Build history of the part. All positions in model axes, mm. Give positions to 0.01 mm unless a question says otherwise; leave off trailing zeros. Order: outer loops, then holes, each group sorted by start corner. A loop starts at its lowest first (then second) coordinate and runs counter-clockwise, first axis right, second up. Notation, with made-up numbers: M 25.25,-36.5 L 31.25,-36.5 A23 cw 31.25,-4.5 Z; hole C -2,-27 d6. An arc over 180 degrees is marked long. One line per item, written item: value.
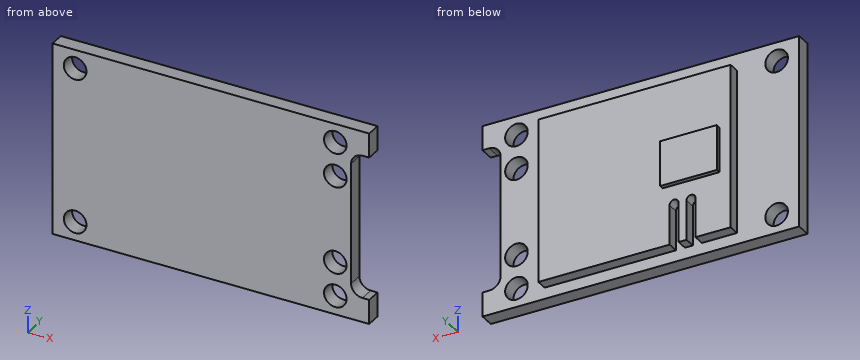
from build123d import *

# Parameters (mm, degrees)
EXTRUDE_1_DEPTH     = 1.3
SKETCH_2_R          = 1
CUT_EXTRUDE_1_DEPTH = 17.429850882
EXTRUDE_2_DEPTH     = 1
SKETCH_4_W          = 5
SKETCH_4_H          = 4
EXTRUDE_3_DEPTH     = 0.4


with BuildPart() as part:
    # Эскиз1 → Бобышка-Вытянуть1 (new body)
    with BuildSketch(Plane(origin=(0, 0, 0), x_dir=(1, 0, 0), z_dir=(0, 1, 0))):
        with BuildLine():
            Line((12.4, 5.35), (12.4, -5.35))
            ThreePointArc((12.4, -5.35), (12.692893219, -6.057106781), (13.4, -6.35))
            Line((13.4, -6.35), (14, -6.35))
            Line((14, -6.35), (14, -8.5))
            Line((14, -8.5), (-14, -8.5))
            Line((-14, -8.5), (-14, 8.5))
            Line((-14, 8.5), (14, 8.5))
            Line((14, 8.5), (14, 6.35))
            Line((14, 6.35), (13.4, 6.35))
            ThreePointArc((13.4, 6.35), (12.692893219, 6.057106781), (12.4, 5.35))
        make_face()
    extrude(amount=EXTRUDE_1_DEPTH)

    # Эскиз2 → Вырез-Вытянуть1 (cut, through all)
    with BuildSketch(Plane(origin=(0, 1.3, 0), x_dir=(1, 0, 0), z_dir=(0, 1, 0))):
        with Locations(Location((11, 6.85, 0), (0, 0, 270))):
            Circle(SKETCH_2_R)
        with Locations(Location((-12, 6.85, 0), (0, 0, 270))):
            Circle(SKETCH_2_R)
        with Locations(Location((-12, -6.85, 0), (0, 0, 270))):
            Circle(SKETCH_2_R)
        with Locations(Location((11, -6.85, 0), (0, 0, 270))):
            Circle(SKETCH_2_R)
        with Locations(Location((11, -3.85, 0), (0, 0, 270))):
            Circle(SKETCH_2_R)
        with Locations(Location((11, 3.85, 0), (0, 0, 270))):
            Circle(SKETCH_2_R)
    extrude(amount=-CUT_EXTRUDE_1_DEPTH, mode=Mode.SUBTRACT)

    # Эскиз3 → Бобышка-Вытянуть2 (add)
    with BuildSketch(Plane(origin=(0, 1.3, 0), x_dir=(1, 0, 0), z_dir=(0, 1, 0))):
        with BuildLine():
            Line((-5.4, 4), (-5.4, 7.5))
            Line((-5.4, 7.5), (-8.5, 7.5))
            Line((-8.5, 7.5), (-8.5, -7))
            Line((-8.5, -7), (8.5, -7))
            Line((8.5, -7), (8.5, 7.5))
            Line((8.5, 7.5), (-3.1, 7.5))
            Line((-3.1, 7.5), (-3.1, 4))
            ThreePointArc((-3.1, 4), (-3.5, 3.6), (-3.9, 4))
            Line((-3.9, 4), (-3.9, 7.5))
            Line((-3.9, 7.5), (-4.6, 7.5))
            Line((-4.6, 7.5), (-4.6, 4))
            ThreePointArc((-4.6, 4), (-5, 3.6), (-5.4, 4))
        make_face()
    extrude(amount=EXTRUDE_2_DEPTH)

    # Эскиз4 → Бобышка-Вытянуть3 (add)
    with BuildSketch(Plane(origin=(0, 2.3, 0), x_dir=(1, 0, 0), z_dir=(0, 1, 0))):
        with Locations((-5, 0.3)):
            Rectangle(SKETCH_4_W, SKETCH_4_H)
    extrude(amount=EXTRUDE_3_DEPTH)


solid = part.part
1) Saw through at A-A, the plane x = -12. Write the cut outline in (y, z).
Check values:
outline: M 0,-8.5 L 1.3,-8.5 L 1.3,-7.85 L 0,-7.85 Z; M 0,-5.85 L 1.3,-5.85 L 1.3,5.85 L 0,5.85 Z; M 0,7.85 L 1.3,7.85 L 1.3,8.5 L 0,8.5 Z
2) Saw through at B-B, the plane z = 3.25. Write the cut outline in (x, y).
Check values:
outline: M -14,0 L 10.2,0 L 10.2,1.3 L 8.5,1.3 L 8.5,2.3 L -8.5,2.3 L -8.5,1.3 L -14,1.3 Z; M 11.8,0 L 12.4,0 L 12.4,1.3 L 11.8,1.3 Z
3) Pin check, flat tips, straight feed: pin 1 (1.2 mm diameter, centred on x = 11, z = -3.85, fed in from +Y); pin 2 (0.8 mm diameter, centred on y = 2, z = -6.5, fed in from -X); pin 3 (0.8 mm diameter, centred on y = 1.5, z = -2, fed in from +X); pin 4 (3 mm diameter, centred on x = 11, z = 3.85, fed in from +Y). Stop position of each tip, or through.
Check values:
pin 1: through
pin 2: x = -8.5
pin 3: x = 12.4
pin 4: y = 1.3
4) Saw through at D-D, the plane x = 11. Write the cut outline in (y, z), then the cut area to 3 significant figures.
Check values:
outline: M 0,-8.5 L 1.3,-8.5 L 1.3,-7.85 L 0,-7.85 Z; M 0,-5.85 L 1.3,-5.85 L 1.3,-4.85 L 0,-4.85 Z; M 0,-2.85 L 1.3,-2.85 L 1.3,2.85 L 0,2.85 Z; M 0,4.85 L 1.3,4.85 L 1.3,5.85 L 0,5.85 Z; M 0,7.85 L 1.3,7.85 L 1.3,8.5 L 0,8.5 Z
area: 11.7 mm^2
5) Saw through at C-C, the plane y = 0.5. Write the cut outline in (x, z).
Check values:
outline: M -14,-8.5 L 14,-8.5 L 14,-6.35 L 13.4,-6.35 A1 cw 12.4,-5.35 L 12.4,5.35 A1 cw 13.4,6.35 L 14,6.35 L 14,8.5 L -14,8.5 Z; hole C -12,-6.85 d2; hole C -12,6.85 d2; hole C 11,-6.85 d2; hole C 11,-3.85 d2; hole C 11,3.85 d2; hole C 11,6.85 d2
6) Drill centre lines: probe 1 along X at (y, z) = (1.35, -7.25); probe 2 along X at (y, z) = (0.65, -6.85); probe 3 along X at (y, z) = (0.65, 3.85). Where is each one in solid material? Low to high. Write a range as from..to.
Check values:
probe 1: -8.5..-5.4, -4.6..-3.9, -3.1..8.5
probe 2: -14..-13, -11..10, 12..14
probe 3: -14..10, 12..12.4
